Source: CAD feature listing. Evaluate the final solid. Frame: model axes, mm. A direction names the side the tool comes from. Round coordinates to 2 decimals unless told otherwise and drop trailing zeros. Loops run counter-clockwise (first coordinate to the right, second up) from the corner with the lowest first, then second, coordinate; pieces in that order, holes last. Notation, with made-up numbers: (-19.5, 62) - (28.5, 62) arc R14 ccw to (28.5, 81) - close; hole circle Ø11 at (15, 53.25). An arc over 180 degrees is marked (long way). One line per question, with ' | ' between items. Start each with the question number.
1. Cut plane B-B (y = -6.25). Return loops of the section in (x, z).
2. Cut plane C-C (z = 52). Return loops of the section in (x, y), then the cut area to 3 significant figures.
3. Pin query (flat end, axial travel): pin 1 (12 mm diameter, centred on x = 9.5, z = 63, fed in from -Y); pin 2 (3.5 mm diameter, centred on x = 0, z = -2.5, fed in from -Y); pin 3 (6.5 mm diameter, centred on x = 1, y = 12.5, fed in from -Z). Return the tip coordinate at first contact, or that it passes through.
4. Ray query, line 1 (Z direction, x = -2, y = -6.5); line 2 (Z direction, x = 3, y = -6.75); line 3 (Z direction, x = 8.25, y = -3.5). Return the intervals inside material, ascending.
5. Mould query, pull axis X, two halves, no side actions, for faces 1 (the flat face through (3, -3, 50.5)), 2 (the cylindrical face through (-11.99, -0.53, 15.78)), 3 (the cylindrical face through (-9.5, 0.07, 48.04)), 4 (the flat face through (7, 12, -2)). Classes: pulls with the +X half, pulls with the -X half, needs draft (parallel to the pull), parting line crosses it, or undercut.
6. Cut plane A-A (x = 0). Return loops of the section in (y, z).
7. Access query for faces 5 (the cylindrical face through (3.233, 1.341, 51.979)), 6 (the flat face through (0, 12, -4.5)), 7 (the cylindrical face through (-6.466, 2.681, -2.958)), 8 (the flat face through (0, 9, -2)). Directions: +Z, -Z, +X, -X, +Y, -Y. A direction counts if a zero-diameter tool reaches every point of the face in a straight line with its end or side. Return the directions, or none.
Autodesk Inventor part; units mm, degrees
ref_plane "YZ Plane" through (0, 0, 0) normal (1, 0, 0) x (0, 1, 0)
ref_plane "XZ Plane" through (0, 0, 0) normal (0, 1, 0) x (-1, 0, 0)
ref_plane "XY Plane" through (0, 0, 0) normal (0, 0, 1) x (1, 0, 0)
sketch "Sketch1" plane through (0, 0, 0) normal (0, 0, 1) x (1, 0, 0)
  circle A0 centre (0, 0) radius 12
  dimension "d0" = 24
extrude "Extrusion1" add sketch "Sketch1" along normal blind 32
sketch "Sketch2" plane through (0, 0, 32) normal (0, 0, 1) x (1, 0, 0)
  circle A0 centre (0, 0) radius 12.5
  dimension "d3" = 25
sketch "Sketch3" plane through (0, 0, 32) normal (0, 0, 1) x (1, 0, 0)
  point P0 (0, 0)
extrude "Extrusion2" add sketch "Sketch2" along normal blind 18.5
sketch "Sketch4" plane through (0, 0, 50.5) normal (0, 0, 1) x (1, 0, 0)
  circle A0 centre (0, 0) radius 3.5
  dimension "d6" = 7
extrude "Extrusion3" add sketch "Sketch4" along normal blind 3
sketch "Sketch7" plane through (0, 0, 0) normal (0, 0, -1) x (-1, 0, 0)
  circle A0 centre (0, 0) radius 7
  dimension "d15" = 14
extrude "Extrusion6" add sketch "Sketch7" along normal blind 6
sketch "Sketch8" plane through (0, 0, 0) normal (0, 0, -1) x (-1, 0, 0)
  circle A0 centre (0, 0) radius 12
  line L0 (0, 9) -> (7, 9)
  line L1 (7, 9) -> (7, 15)
  line L2 (7, 15) -> (-7, 15)
  line L3 (-7, 15) -> (-7, 9)
  line L4 (-7, 9) -> (0, 9)
  dimension "d20" = 7
  dimension "d21" = 14
extrude "Extrusion7" add sketch "Sketch8" along normal blind 4.5 contours L1 L0 L4 L3 A0 | A0 L3 L2 L1 picked at (-3.7936, 9.7239)
sketch "Sketch9" plane through (0, 0, 50.5) normal (0, 0, 1) x (1, 0, 0)
  circle A0 centre (-8, 0) radius 1.5
  circle A1 centre (8, 0) radius 1.5
  point P0 (0, 0)
  dimension "d24" = 3
  dimension "d25" = 8
  dimension "d26" = 3
  dimension "d27" = 8
extrude "Extrusion8" cut sketch "Sketch9" against normal blind 5
sketch "Sketch10" plane through (0, 0, 53.5) normal (0, 0, 1) x (1, 0, 0)
  circle A0 centre (0, 0) radius 4
  dimension "d30" = 8
extrude "Extrusion9" add sketch "Sketch10" along normal blind 12
sketch "Sketch11" plane through (0, 0, 65.5) normal (0, 0, 1) x (1, 0, 0)
  circle A0 centre (0, 0) radius 7
  circle A1 centre (0, 0) radius 8
  dimension "d33" = 16
extrude "Extrusion10" add sketch "Sketch11" along normal blind 8 contours A0 | A1
properties part number "Motor_Place_Holder"
Answers follow:
1) outline: (-10.83, 32) - (-10.24, 32) - (-10.24, 0) - (-3.15, 0) - (-3.15, -6) - (3.15, -6) - (3.15, 0) - (10.24, 0) - (10.24, 32) - (10.83, 32) - (10.83, 50.5) - (-10.83, 50.5) - close; (-4.99, 65.5) - (4.99, 65.5) - (4.99, 73.5) - (-4.99, 73.5) - close
2) outline: circle Ø7 at (0, 0) | area: 38.5 mm2
3) pin 1: stops at y = -6.9 | pin 2: stops at y = -7 | pin 3: stops at z = -4.5
4) line 1: z = -6 to 50.5, 65.5 to 73.5 | line 2: z = 0 to 50.5, 65.5 to 73.5 | line 3: z = 0 to 50.5
5) face 1: needs draft | face 2: parting line crosses it | face 3: undercut | face 4: pulls with the +X half
6) outline: (-12.5, 32) - (-12, 32) - (-12, 0) - (-7, 0) - (-7, -6) - (7, -6) - (7, 0) - (9, 0) - (9, -4.5) - (15, -4.5) - (15, 0) - (12, 0) - (12, 32) - (12.5, 32) - (12.5, 50.5) - (3.5, 50.5) - (3.5, 53.5) - (4, 53.5) - (4, 65.5) - (8, 65.5) - (8, 73.5) - (-8, 73.5) - (-8, 65.5) - (-4, 65.5) - (-4, 53.5) - (-3.5, 53.5) - (-3.5, 50.5) - (-12.5, 50.5) - close
7) face 5: none | face 6: -Z, +X, -X, +Y | face 7: -Z | face 8: -Z, +X, -X
